Source: CAD feature listing. Evaluate the final solid. Frame: model axes, mm. Face numbers are marked on the shaded views. A direction names the side the tool comes from. Give positions to 0.01 mm unless a question says otherwise; leave off trailing zeros. Order: outer loops, then holes, each group sorted by start corner. A loop starts at its lowest first (then second) coordinate and runs counter-clockwise, first axis right, second up.
```python
from build123d import *

# Parameters (mm, degrees)
SKETCH1_W           = 45
SKETCH1_H           = 50.7
SKETCH1_R           = 2.636973336
SKETCH1_R_2         = 3.554118364
SKETCH1_R_3         = 2.989089767
BOSS_EXTRUDE1_DEPTH = 2
SKETCH2_W           = 30.94366189
SKETCH2_H           = 37.292040818
BOSS_EXTRUDE2_DEPTH = 35


with BuildPart() as part:
    # Sketch1 → Boss-Extrude1 (new body)
    with BuildSketch(Plane.XY):
        Rectangle(SKETCH1_W, SKETCH1_H)
        with Locations((0, 15.621214427)):
            Circle(SKETCH1_R, mode=Mode.SUBTRACT)
        with Locations((-12.932898819, 5.05104632)):
            Circle(SKETCH1_R_2, mode=Mode.SUBTRACT)
        with Locations((-9.047478573, -11.600754735)):
            Circle(SKETCH1_R_3, mode=Mode.SUBTRACT)
        with Locations((9.047478573, -11.600754735)):
            Circle(SKETCH1_R_3, mode=Mode.SUBTRACT)
        with Locations((12.932898819, 5.05104632)):
            Circle(SKETCH1_R_2, mode=Mode.SUBTRACT)
    extrude(amount=BOSS_EXTRUDE1_DEPTH)

    # Sketch2 → Boss-Extrude2 (add)
    with BuildSketch(Plane.XY.offset(2)):
        Rectangle(SKETCH2_W, SKETCH2_H)
    extrude(amount=BOSS_EXTRUDE2_DEPTH)


solid = part.part
```
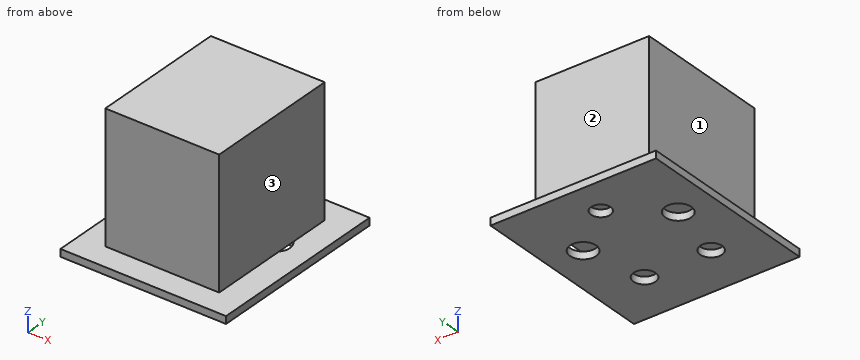
1) Section query C-C, the plane z = 22. Return the cut outline in (x, y), and give its area (3 significant figures).
Report:
outline: (-15.47, -18.65) - (15.47, -18.65) - (15.47, 18.65) - (-15.47, 18.65) - close
area: 1,150 mm2
2) Pin query (flat end, axial travel): pin 1 (4 mm diameter, centred on x = 9.5, z = 31, fed in from -Y); pin 2 (2 mm diameter, centred on x = -5, z = 14.5, fed in from +Y); pin 3 (1.8 mm diameter, centred on x = 12, y = 4.5, fed in from -Z). Return the tip coordinate at first contact, or that it passes through.
Report:
pin 1: stops at y = -18.65
pin 2: stops at y = 18.65
pin 3: stops at z = 2
3) Reachability of the marked faces 1, 2 and 3 from +Z, -Z, +X, -X, +Y, -Y: full face, straight path, thin tool, end or side. Return the list, or none.
Report:
face 1: +Z, -X, +Y, -Y
face 2: +Z, +X, -X, +Y
face 3: +Z, +X, +Y, -Y
4) Material intervals for L1, parallel to Y at x = 0, z = 1.65; L2, parallel to Y at x = 3, z = 7.5; L3, parallel to X at y = -11, z = 4.5, sorted ascending.
Report:
L1: y = -25.35 to 12.98, 18.26 to 25.35
L2: y = -18.65 to 18.65
L3: x = -15.47 to 15.47
5) Section query D-D, the plane x = -11. Return the cut outline in (y, z), and give its area (3 significant figures).
Report:
outline: (-25.35, 0) - (-13.86, 0) - (-13.86, 2) - (-9.34, 2) - (-9.34, 0) - (2.07, 0) - (2.07, 2) - (8.03, 2) - (8.03, 0) - (25.35, 0) - (25.35, 2) - (18.65, 2) - (18.65, 37) - (-18.65, 37) - (-18.65, 2) - (-25.35, 2) - close
area: 1,390 mm2
6) Section query B-B, the plane y = -18. Return the cut outline in (x, z), and give its area (3 significant figures).
Report:
outline: (-22.5, 0) - (22.5, 0) - (22.5, 2) - (15.47, 2) - (15.47, 37) - (-15.47, 37) - (-15.47, 2) - (-22.5, 2) - close
area: 1,170 mm2
7) Section query A-A, the plane x = 0. Return the cut outline in (y, z), and give its area (3 significant figures).
Report:
outline: (-25.35, 0) - (12.98, 0) - (12.98, 2) - (18.26, 2) - (18.26, 0) - (25.35, 0) - (25.35, 2) - (18.65, 2) - (18.65, 37) - (-18.65, 37) - (-18.65, 2) - (-25.35, 2) - close
area: 1,400 mm2
